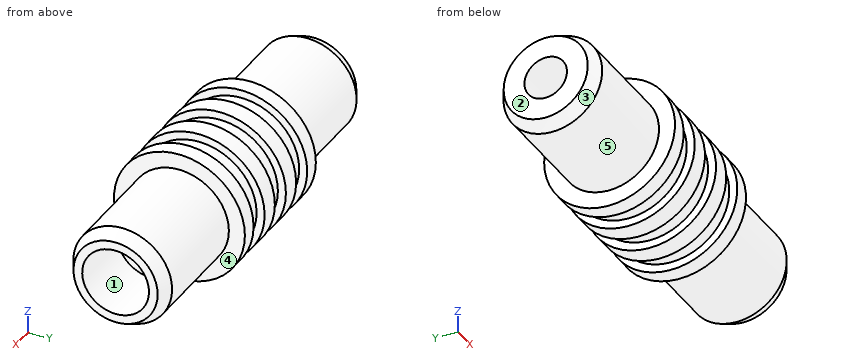
```python
from build123d import *

# Parameters (mm, degrees)
SKETCH2_W          = 1.9812
SKETCH2_H          = 1.524
SKETCH3_R          = 3.175
CUT_EXTRUDE1_DEPTH = 6.2992


with BuildPart() as part:
    # Sketch1 → Revolve1 (revolve)
    with BuildSketch(Plane.XY):
        Polygon((0, 2.0193), (17.78, 2.0193), (17.78, 4.0005), (16.51, 4.699), (6.35, 4.699), (6.35, 6.223), (0, 6.223), align=None)
    revolve1 = revolve(axis=Axis((0, 0, 0), (1, 0, 0)))

    # Mirror1: Revolve1 across plane
    add(revolve1.mirror(Plane(origin=(0, 6.223, 0), x_dir=(0, 0, 1), z_dir=(1, 0, 0))))

    # Sketch2 → Cut-Revolve1 (revolve, cut)
    with BuildSketch(Plane.XY):
        with Locations((0, 6.223)):
            Rectangle(SKETCH2_W, SKETCH2_H)
        with Locations((-3.81, 6.223)):
            Rectangle(SKETCH2_W, SKETCH2_H)
        with Locations((3.81, 6.223)):
            Rectangle(SKETCH2_W, SKETCH2_H)
    revolve(axis=Axis((0, 0, 0), (1, 0, 0)), mode=Mode.SUBTRACT)

    # Sketch3 → Cut-Extrude1 (cut)
    with BuildSketch(Plane(origin=(17.78, 0, 0), x_dir=(0, 0, -1), z_dir=(1, 0, 0))):
        Circle(SKETCH3_R)
    extrude(amount=-CUT_EXTRUDE1_DEPTH, mode=Mode.SUBTRACT)


solid = part.part
```
Could you check a few things on this model? Use its own coordinates, in mm. Face numbers are marked on the shaded views. A direction names the side the tool comes from. Round coordinates to 2 decimals unless told otherwise and drop trailing zeros. Loops run counter-clockwise (first coordinate to the right, second up) from the corner with the lowest first, then second, coordinate; pieces in that order, holes last. Notation, with made-up numbers: (25, 60) -> (83, 60) arc R30 cw to (83, 85) -> close; hole circle Ø3 at (79, 11.25). An arc over 180 degrees is marked (long way). Put each result on its own line as item: value.
Q1. I want a section at A-A on x = 16. Write out the boundary of the cut face in (y, z) (3 decimals).
Checks:
outline: circle Ø9.398 at (0, 0); hole circle Ø6.35 at (0, 0)
Q2. Which directions (+Z, -Z, +X, -X, +Y, -Y) give clear straight access to the entire face, cutting with the end or side of a thin tool? Please do the marked faces 4 and 5.
Checks:
face 4: +X
face 5: -X
Q3. Thinking about a two-plate mould opening in Z: for the marked faces 1, 2 and 3, which applies, pulls with the +Z half, pulls with the -Z half, needs draft (parallel to the pull), parting line crosses it, or undercut?
Checks:
face 1: undercut
face 2: needs draft
face 3: parting line crosses it
Q4. Please list where these lines run through material, in increasing order: line 1 (X direction, y = -1.5, z = 5.5); line 2 (Z direction, x = -7, y = 0); line 3 (Z direction, x = 4, y = 0). Write a range as from..to.
Checks:
line 1: -6.35..-4.8, -2.82..-0.99, 0.99..2.82, 4.8..6.35
line 2: -4.7..-2.02, 2.02..4.7
line 3: -5.46..-2.02, 2.02..5.46
Q5. I want a section at B-B on x = -12.5. Write out the boundary of the cut face in (y, z), and give its area (3 significant figures).
Checks:
outline: circle Ø9.4 at (0, 0); hole circle Ø4.04 at (0, 0)
area: 56.6 mm2
Q6. For pin 1 Ø3 at (x, y) = (-7.5, 3) entering from +Z; pin 2 Ø1.9 at (y, z) = (1, -1) entering from +X; pin 3 Ø1 at (x, y) = (0, -5) entering from +Z; pin 4 Ø6 at (y, z) = (-1, -1) entering from +X, each with a flat end and sliding along its axis, tell me the tip position at first contact or that it passes through.
Checks:
pin 1: z = 5.88
pin 2: x = 11.48
pin 3: z = 3.09
pin 4: x = 17.78
